```python
from build123d import *

# Parameters (mm, degrees)
F0_R     = 12.7
F1_DEPTH = 9.652


with BuildPart() as f1:
    # F0 (on Top) → F1 (new body)
    with BuildSketch(Plane.XY):
        with BuildLine():
            Line((-71.649214, 0), (-65.185605, 0))
            Line((-65.185605, 0), (-65.185605, -96.52))
            Line((-65.185605, -96.52), (-14.385605, -96.52))
            Line((-14.385605, -96.52), (-14.385605, 0))
            Line((-14.385605, 0), (0, 0))
            ThreePointArc((0, 0), (-153.784762, 158.779921), (-268.724012, -30.031586))
            Line((-268.724012, -30.031586), (-220.815669, 0))
            ThreePointArc((-220.815669, 0), (-213.330935, 6.066045), (-208.444798, 14.369287))
            Line((-208.444798, 14.369287), (-160.438798, 14.369287))
            ThreePointArc((-160.438798, 14.369287), (-138.269006, -2.915778), (-116.099214, 14.369287))
            Line((-116.099214, 14.369287), (-71.649214, 14.369287))
            Line((-71.649214, 14.369287), (-71.649214, 0))
        make_face()
        with Locations((-233.844798, 23.726932)):
            Circle(F0_R, mode=Mode.SUBTRACT)
        with Locations((-138.269006, 19.944222)):
            Circle(F0_R, mode=Mode.SUBTRACT)
        with Locations((-42.693214, 23.726932)):
            Circle(F0_R, mode=Mode.SUBTRACT)
        with Locations((-204.553327, 88.903846)):
            Circle(F0_R, mode=Mode.SUBTRACT)
        with Locations((-71.984685, 88.903846)):
            Circle(F0_R, mode=Mode.SUBTRACT)
        with Locations((-138.269006, 115.594841)):
            Circle(F0_R, mode=Mode.SUBTRACT)
    extrude(amount=F1_DEPTH)


solid = f1.part
```
The model under review builds one solid part; all positions refer to its coordinate system, in mm. A direction names the side the tool comes from. Coordinates: 2 decimals unless noted, no trailing zeros. Loops run counter-clockwise (first coordinate to the right, second up) from the corner with the lowest first, then second, coordinate; pieces in that order, holes last. Notation, with made-up numbers: (85.25, 34.5) -> (111.25, 34.5) arc R4 cw to (111.25, 40.5) -> close; hole circle Ø4 at (77.25, 50). An arc over 180 degrees is marked (long way). Answer as CSV lines item,"result".
Item 1: Machinability: for faces 4 (the flat face through (-140, 62, 9.652)), 5 (the flat face through (-245.11, -15.23, 4.76)), 6 (the flat face through (-14.386, -49, 5)), which of the approach directions +Z, -Z, +X, -X, +Y, -Y give a long, thin tool a straight path to every point of the face, cutting with its end or side? Answer none if there is none.
Results below:
face 4,"+Z, +X, -X, +Y, -Y"
face 5,"+Z, -Z, -Y"
face 6,"+Z, -Z, +X, -Y"
Item 2: Take a section at D-D, the plane y = -69.5. State the section outline as (x, z) points, and give its area (3 significant figures).
Results below:
outline,"(-65.19, 0) -> (-14.39, 0) -> (-14.39, 9.65) -> (-65.19, 9.65) -> close"
area,"490 mm2"
Item 3: Insertion check: pin 1 (1.5 mm diameter, centred on x = -71.5, z = 6.5, fed in from -Y); pin 2 (5 mm diameter, centred on x = -181, z = 6, fed in from -Y); pin 3 (23 mm diameter, centred on x = -138.27, y = 115.59, fed in from +Z); pin 4 (1 mm diameter, centred on x = -214, z = 6, fed in from +Y). Each pin has a flat end and moves straight along its axis. Give the tip position at first contact, or say it passes through.
Results below:
pin 1,"stops at y = 0"
pin 2,"stops at y = 14.37"
pin 3,"passes through"
pin 4,"stops at y = 137.66"
Item 4: Take a section at C-C, the plane z = 8. State the section outline as (x, y) points.
Results below:
outline,"(-268.72, -30.03) -> (-220.82, 0) arc R27.07 ccw to (-208.44, 14.37) -> (-160.44, 14.37) arc R22.86 ccw to (-116.1, 14.37) -> (-71.65, 14.37) -> (-71.65, 0) -> (-65.19, 0) -> (-65.19, -96.52) -> (-14.39, -96.52) -> (-14.39, 0) -> (0, 0) arc R139.7 ccw (long way) to start; hole circle Ø25.4 at (-233.84, 23.73); hole circle Ø25.4 at (-204.55, 88.9); hole circle Ø25.4 at (-138.27, 19.94); hole circle Ø25.4 at (-138.27, 115.59); hole circle Ø25.4 at (-71.98, 88.9); hole circle Ø25.4 at (-42.69, 23.73)"
Item 5: Take a section at B-B, the plane x = -44. State the section outline as (y, z) points, and give its area (3 significant figures).
Results below:
outline,"(-96.52, 0) -> (11.09, 0) -> (11.09, 9.65) -> (-96.52, 9.65) -> close; (36.36, 0) -> (123.04, 0) -> (123.04, 9.65) -> (36.36, 9.65) -> close"
area,"1,880 mm2"
Item 6: For L1, parallel to Y at x = -143, z = 1; L2, parallel to X at y = 81.5, z = 7.25; L3, parallel to X at y = 99.5, z = 0.5, list the stretches that pass through material, from the lowest coordinate up.
Results below:
L1,"y = -2.42 to 8.16, 31.73 to 103.81, 127.38 to 159.56"
L2,"x = -263.68 to -214.87, -194.23 to -82.3, -61.67 to -12.86"
L3,"x = -253.1 to -211.55, -197.55 to -78.99, -64.98 to -23.43"
Item 7: Draft analysis for pull direction X (two halves, no side actions). For faces 1 (the flat face through (-140, 62, 0)), 2 (the cylindrical face through (-150.23, 159.13, 4.76)), 3 (the cylindrical face through (-213.9, 97.5, 4.8)), state which applies: +X half, -X half, draft (parallel to the pull), parting line (faces both ways), or undercut.
Results below:
face 1,"draft"
face 2,"parting line"
face 3,"undercut"
Item 8: Take a section at A-A, the plane y = -26.5. State the section outline as (x, z) points, and give its area (3 significant figures).
Results below:
outline,"(-270.02, 0) -> (-263.09, 0) -> (-263.09, 9.65) -> (-270.02, 9.65) -> close; (-65.19, 0) -> (-14.39, 0) -> (-14.39, 9.65) -> (-65.19, 9.65) -> close"
area,"557 mm2"
